Here's how the part is built. I have some questions about the finished solid (model axes, mm). A direction names the side the tool comes from. Round coordinates to 2 decimals unless told otherwise and drop trailing zeros. Write each loop counter-clockwise with the first axis right and the second up, starting at its lowest first coordinate (ties: lowest second). Pieces come first, ordered by that corner, then holes. Notation, with made-up numbers: M -19.5,67.5 L -12.5,67.5 A12 cw -12.5,78.5 Z; hole C 60,10 d7. An arc over 180 degrees is marked long. Use one line per item in the form item = value. Start each with the question number.
Q1. I want a section at A-A on y = 23. List the corners of the cut face in (x, z) for me.
Q2. I want a section at C-C on z = 36.5. List the corners of the cut face in (x, y) for me, and give its area (3 significant figures).
Q3. For faces 1 (the face through (0, 30, -1)), 2 (the face through (0, -27.7, -2)), which set-ups out of +Z, -Z, +X, -X, +Y, -Y let a thin tool reach every point of the face, with its end or its side?
Q4. I want a section at D-D on x = -15. List the corners of the cut face in (y, z) for me, and give its area (3 significant figures).
Q5. I need wall thicknesses on line 1 along Y through (x, z) = (-16.5, 13); line 2 along X through (y, z) = (7, -58); line 3 along Y through (x, z) = (3, 64). Which ranges of each line are inside material? Lowest first, please. Write a range as from..to.
Q6. We'd pull the mould along Y, two halves only. Please class faces 3 (the face through (-18, 0, 80)), 4 (the face through (-20, -7, -2)), 5 (the face through (0, -30, -2)), 6 (the face through (-17.7, -6, -2)): +Y half, -Y half, draft (parallel to the pull), parting line (faces both ways), or undercut.
Q7. I'm going to push a flat-ended pin straight in: pin 1 Ø14.5 at (x, z) = (0, 25) entering from -Y. Where does the tip first touch, or does it pass through?
Q8. I want a section at B-B on x = 0. List the corners of the cut face in (y, z) for me.
Autodesk Inventor part; units mm, degrees
ref_plane "YZ Plane" through (0, 0, 0) normal (1, 0, 0) x (0, 1, 0)
ref_plane "XZ Plane" through (0, 0, 0) normal (0, 1, 0) x (-1, 0, 0)
ref_plane "XY Plane" through (0, 0, 0) normal (0, 0, 1) x (1, 0, 0)
sketch "スケッチ1" plane through (0, 0, 0) normal (0, 0, 1) x (1, 0, 0)
  line L0 (-20, 30) -> (20, 30)
  line L1 (20, 30) -> (20, -30)
  line L2 (20, -30) -> (-20, -30)
  line L3 (-20, -30) -> (-20, 30)
  line L4 (-20, 30) -> (20, -30) construction
  line L5 (20, 30) -> (-20, -30) construction
  line L6 (17.7, 27.7) -> (-17.7, 27.7)
  line L7 (-17.7, 27.7) -> (-17.7, -27.7)
  line L8 (-17.7, -27.7) -> (17.7, -27.7)
  line L9 (17.7, -27.7) -> (17.7, 27.7)
  point P0 (0, 0)
  dimension "d0" = 40
  dimension "d1" = 60
  dimension "d2" = 2.3
extrude "押し出し1" add sketch "スケッチ1" along normal mid plane 220
chamfer "面取り1" distance 60 angle 45 2 edges at (0, 30, 110) (0, 30, -110)
sketch "スケッチ5" plane through (-20, -30, 110) normal (0, -1, 0) x (1, 0, 0)
  circle A0 centre (20, -85) radius 6.25
  point P0 (20, -110)
  dimension "d14" = 12.5
  dimension "d17" = 25
extrude "押し出し3" cut sketch "スケッチ5" against normal blind 250
properties part number "車軸受け1"
Reported:
q1.outline = M -20,-57 L -17.7,-57 L -17.7,57 L -20,57 Z; M 17.7,-57 L 20,-57 L 20,57 L 17.7,57 Z
q2.outline = M -20,-30 L 20,-30 L 20,30 L -20,30 Z; hole M -17.7,-27.7 L 17.7,-27.7 L 17.7,27.7 L -17.7,27.7 Z
q2.area = 439 mm^2
q3.face_1 = +Z, -Z, +X, -X, +Y
q3.face_2 = +Z, -Z
q4.outline = M -30,-110 L -27.7,-107.7 L -27.7,107.7 L -30,110 Z; M 27.7,-52.3 L 30,-50 L 30,50 L 27.7,52.3 Z
q4.area = 736 mm^2
q5.line_1 = -30..-27.7, 27.7..30
q5.line_2 = -20..-17.7, 17.7..20
q5.line_3 = -30..-27.7
q6.face_3 = +Y half
q6.face_4 = draft
q6.face_5 = -Y half
q6.face_6 = undercut
q7.pin_1 = -30
q8.outline = M -30,-110 L -27.7,-107.7 L -27.7,18.75 L -30,18.75 Z; M -30,31.25 L -27.7,31.25 L -27.7,107.7 L -30,110 Z; M 27.7,-52.3 L 30,-50 L 30,18.75 L 27.7,18.75 Z; M 27.7,31.25 L 30,31.25 L 30,50 L 27.7,52.3 Z
